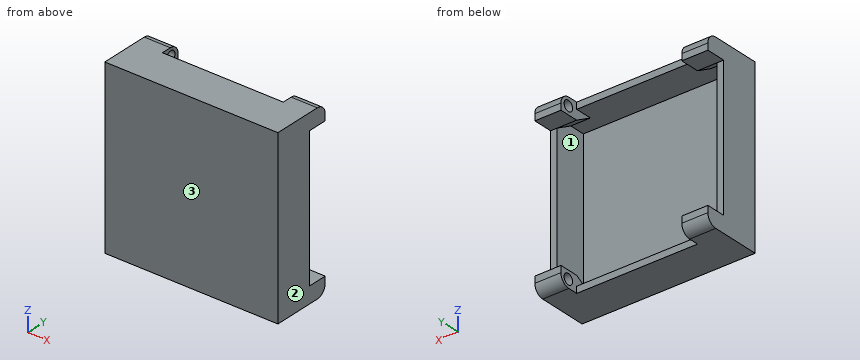
from build123d import *
from OCP.BRepFilletAPI import BRepFilletAPI_MakeChamfer

# Parameters (mm, degrees)
SKETCH1_W               = 53
SKETCH1_H               = 53
SKETCH1_W_2             = 49
SKETCH1_H_2             = 49
BOSS_EXTRUDE1_DEPTH     = 10
SKETCH2_W               = 53
SKETCH2_H               = 53
BOSS_EXTRUDE2_DEPTH     = 2
SKETCH3_W               = 8
SKETCH3_H               = 5
BOSS_EXTRUDE3_DEPTH     = 6
CHAMFER3_SIZE           = 5.196152423
CHAMFER3_SIZE_2         = 3
CUT_EXTRUDE1_DEPTH      = 22
CUT_EXTRUDE1_DEPTH_BACK = 22
SKETCH4_R               = 1.6
FILLET3_R               = 3


with BuildPart() as part:
    # Sketch1 → Boss-Extrude1 (new body)
    with BuildSketch(Plane(origin=(0, 0, 0), x_dir=(1, 0, 0), z_dir=(0, 1, 0))):
        Rectangle(SKETCH1_W, SKETCH1_H)
        Rectangle(SKETCH1_W_2, SKETCH1_H_2, mode=Mode.SUBTRACT)
    extrude(amount=BOSS_EXTRUDE1_DEPTH)

    # Sketch2 → Boss-Extrude2 (add)
    with BuildSketch(Plane.XZ):
        Rectangle(SKETCH2_W, SKETCH2_H)
    extrude(amount=BOSS_EXTRUDE2_DEPTH)

    # Sketch3 → Boss-Extrude3 (add)
    with BuildSketch(Plane(origin=(0, 10, 0), x_dir=(1, 0, 0), z_dir=(0, 1, 0))):
        with Locations((-22.5, -24)):
            Rectangle(SKETCH3_W, SKETCH3_H)
        with Locations((22.5, -24)):
            Rectangle(SKETCH3_W, SKETCH3_H)
        with Locations((22.5, 24)):
            Rectangle(SKETCH3_W, SKETCH3_H)
        with Locations((-22.5, 24)):
            Rectangle(SKETCH3_W, SKETCH3_H)
    extrude(amount=BOSS_EXTRUDE3_DEPTH)

    # Chamfer3
    chamfer3_edges_1 = [part.edges().sort_by_distance(p)[0] for p in [
        (-21.5, 10, -24.5),
    ]]
    chamfer3_side_1 = [part.faces().sort_by_distance(p)[0] for p in [
        (-21.5, 9.94, -24.5),
    ]]
    chamfer3_edges_2 = [part.edges().sort_by_distance(p)[0] for p in [
        (-21.5, 10, 24.5),
    ]]
    chamfer3_side_2 = [part.faces().sort_by_distance(p)[0] for p in [
        (-21.5, 10, 24.44),
    ]]
    chamfer3_edges_3 = [part.edges().sort_by_distance(p)[0] for p in [
        (21.5, 10, 24.5),
    ]]
    chamfer3_side_3 = [part.faces().sort_by_distance(p)[0] for p in [
        (21.5, 9.94, 24.5),
    ]]
    chamfer3_edges_4 = [part.edges().sort_by_distance(p)[0] for p in [
        (21.5, 10, -24.5),
    ]]
    chamfer3_side_4 = [part.faces().sort_by_distance(p)[0] for p in [
        (21.5, 10, -24.44),
    ]]
    chamfer3 = BRepFilletAPI_MakeChamfer(part.part.solid().wrapped)
    for e in chamfer3_edges_1:
        chamfer3.Add(CHAMFER3_SIZE - 0.0001, CHAMFER3_SIZE_2 - 0.0001, e.wrapped, chamfer3_side_1[0].wrapped)
    for e in chamfer3_edges_2:
        chamfer3.Add(CHAMFER3_SIZE_2 - 0.0001, CHAMFER3_SIZE - 0.0001, e.wrapped, chamfer3_side_2[0].wrapped)
    for e in chamfer3_edges_3:
        chamfer3.Add(CHAMFER3_SIZE - 0.0001, CHAMFER3_SIZE_2 - 0.0001, e.wrapped, chamfer3_side_3[0].wrapped)
    for e in chamfer3_edges_4:
        chamfer3.Add(CHAMFER3_SIZE_2 - 0.0001, CHAMFER3_SIZE - 0.0001, e.wrapped, chamfer3_side_4[0].wrapped)
    add(Compound.cast(chamfer3.Shape()), mode=Mode.REPLACE)  # a hair under: the kernel refuses the full size

    # Sketch4 → Cut-Extrude1 (cut, two sides: drawn at the far end of the back side and taken through both)
    with BuildSketch(Plane(origin=(0, 0, 0), x_dir=(0, 0, -1), z_dir=(1, 0, 0)).offset(-CUT_EXTRUDE1_DEPTH_BACK)):
        with Locations((-24, 13.2)):
            Circle(SKETCH4_R)
        with Locations(Location((24, 13.2, 0), (0, 0, 180))):
            Circle(SKETCH4_R)
    extrude(amount=CUT_EXTRUDE1_DEPTH + CUT_EXTRUDE1_DEPTH_BACK, mode=Mode.SUBTRACT)

    # Fillet3
    fillet3_edges = [part.edges().sort_by_distance(p)[0] for p in [
        (-22.5, 16, 26.5),
        (22.5, 16, 26.5),
        (22.5, 16, -26.5),
        (-22.5, 16, -26.5),
    ]]
    fillet(fillet3_edges, radius=FILLET3_R)


solid = part.part
Read the model definition and answer for the solid it produces. Units are mm, in the model's axes. Face numbers are marked on the shaded views. Coordinates: 2 decimals unless noted, no trailing zeros. Order: outer loops, then holes, each group sorted by start corner. A loop starts at its lowest first (then second) coordinate and runs counter-clockwise, first axis right, second up. Notation, with made-up numbers: (-20, -13) -> (35, -13) arc R27 cw to (35, 3) -> close; hole circle Ø7 at (-37.5, 38.25). An arc over 180 degrees is marked (long way). Answer as a JSON object with one key per item and string values.
1) A cutting plane is placed at B-B, the plane z = -9. Determine the outline of the cut face in (x, y).
Model answer:
{"outline": "(-26.5, -2) -> (26.5, -2) -> (26.5, 10) -> (24.5, 10) -> (24.5, 0) -> (-24.5, 0) -> (-24.5, 10) -> (-26.5, 10) -> close"}
2) A cutting plane is placed at C-C, the plane x = 14. Determine the outline of the cut face in (y, z), plus the area to 3 significant figures.
Model answer:
{"outline": "(-2, -26.5) -> (10, -26.5) -> (10, -24.5) -> (0, -24.5) -> (0, 24.5) -> (10, 24.5) -> (10, 26.5) -> (-2, 26.5) -> close", "area": "146 mm²"}
3) Each of these flat-tipped pins is pushed along its axis until it touches: pin 1 (12 mm diameter, centred on x = 2, z = 15, fed in from +Y); pin 2 (1.6 mm diameter, centred on x = 25.5, z = 8.5, fed in from +Y). Where does it stop, or does it pass through?
Model answer:
{"pin 1": "stops at y = 0", "pin 2": "stops at y = 10"}
4) The mould has two halves that part along X. Classify the marked faces 1, 2 and 3: released by +X, released by -X, zero draft, split by the parting line, or undercut.
Model answer:
{"face 1": "undercut", "face 2": "released by +X", "face 3": "zero draft"}
5) Consider line 1 along Z through (x, y) = (19.7, 13.2); line 2 along Z through (x, y) = (2, 0.75). Determine where each line is inside the solid, lowest interval first. Write a range as from..to.
Model answer:
{"line 1": "z = -26.49..-25.6, -22.4..-21.5, 21.5..22.4, 25.6..26.49", "line 2": "z = -26.5..-24.5, 24.5..26.5"}
6) A cutting plane is placed at A-A, the plane y = 1.5. Determine the outline of the cut face in (x, z).
Model answer:
{"outline": "(-26.5, -26.5) -> (26.5, -26.5) -> (26.5, 26.5) -> (-26.5, 26.5) -> close; hole (-24.5, -24.5) -> (24.5, -24.5) -> (24.5, 24.5) -> (-24.5, 24.5) -> close"}
7) A cutting plane is placed at D-D, the plane y = 7. Determine the outline of the cut face in (x, z).
Model answer:
{"outline": "(-26.5, -26.5) -> (26.5, -26.5) -> (26.5, 26.5) -> (-26.5, 26.5) -> close; hole (-24.5, -23.23) -> (-18.5, -23.23) -> (-18.5, -24.5) -> (18.5, -24.5) -> (18.5, -23.23) -> (24.5, -23.23) -> (24.5, 23.23) -> (18.5, 23.23) -> (18.5, 24.5) -> (-18.5, 24.5) -> (-18.5, 23.23) -> (-24.5, 23.23) -> close"}
